CAD build for the part. Positions are in the model's coordinates, mm. Coordinates: 2 decimals unless noted, no trailing zeros. Loops run counter-clockwise (first coordinate to the right, second up) from the corner with the lowest first, then second, coordinate; pieces in that order, holes last. Notation, with made-up numbers: (47.25, -21.75) - (60.25, -21.75) arc R21 cw to (60.25, 6.25) - close; hole circle Ø11 at (12, 64.25). An arc over 180 degrees is marked (long way). Put each result on its own line as item: value.
```python
from build123d import *

# Parameters (mm, degrees)
F0_R     = 11
F1_DEPTH = 9
F2_R     = 1.5
F3_SIZE  = 1


with BuildPart() as f1:
    # F0 (on Top) → F1 (new body)
    with BuildSketch(Plane.XY):
        with BuildLine():
            ThreePointArc((-8.613839, 14.656117), (-15.257844, 12.618509), (-22.107143, 13.793993))
            ThreePointArc((-22.107143, 13.793993), (-43, 0), (-22.107143, -13.793993))
            ThreePointArc((-22.107143, -13.793993), (-15.257844, -12.618509), (-8.613839, -14.656117))
            ThreePointArc((-8.613839, -14.656117), (0, -17), (8.613839, -14.656117))
            ThreePointArc((8.613839, -14.656117), (15.257844, -12.618509), (22.107143, -13.793993))
            ThreePointArc((22.107143, -13.793993), (43, 0), (22.107143, 13.793993))
            ThreePointArc((22.107143, 13.793993), (15.257844, 12.618509), (8.613839, 14.656117))
            ThreePointArc((8.613839, 14.656117), (0, 17), (-8.613839, 14.656117))
        make_face()
        with Locations((-28, 0)):
            Circle(F0_R, mode=Mode.SUBTRACT)
        Circle(F0_R, mode=Mode.SUBTRACT)
        with Locations((28, 0)):
            Circle(F0_R, mode=Mode.SUBTRACT)
    extrude(amount=F1_DEPTH)

    # F2
    f2_edges = [f1.edges().sort_by_distance(p)[0] for p in [
        (0, 17, 0),
        (0, 17, 9),
    ]]
    fillet(f2_edges, radius=F2_R)

    # F3
    f3_edges = [f1.edges().sort_by_distance(p)[0] for p in [
        (-17, 0, 4.5),
        (-39, 0, 0),
        (-39, 0, 9),
        (11, 0, 4.5),
        (-11, 0, 0),
        (-11, 0, 9),
        (39, 0, 4.5),
        (17, 0, 0),
        (17, 0, 9),
    ]]
    chamfer(f3_edges, length=F3_SIZE)


solid = f1.part
```
Q1. Slice it at C-C, the plane y = -6. State how many separate pieces and enclosed holes the cut face has, then the cut area to 3 significant figures.
Determined:
separate pieces: 4
enclosed holes: 0
area: 244 mm2
Q2. Slice it at A-A, the plane x = 0. Give the cut face in (y, z), then the cut area to 3 significant figures.
Determined:
outline: (-17, 1.5) arc R1.5 ccw to (-15.5, 0) - (-12, 0) - (-11, 1) - (-11, 8) - (-12, 9) - (-15.5, 9) arc R1.5 ccw to (-17, 7.5) - close; (11, 1) - (12, 0) - (15.5, 0) arc R1.5 ccw to (17, 1.5) - (17, 7.5) arc R1.5 ccw to (15.5, 9) - (12, 9) - (11, 8) - close
area: 104 mm2
Q3. Slice it at B-B, the plane z = 2.25. Give the cut face in (x, y).
Determined:
outline: (-22.11, -13.79) arc R15 cw to (-8.61, -14.66) arc R17 ccw to (8.61, -14.66) arc R15 cw to (22.11, -13.79) arc R15 ccw (long way) to (22.11, 13.79) arc R15 cw to (8.61, 14.66) arc R17 ccw to (-8.61, 14.66) arc R15 cw to (-22.11, 13.79) arc R15 ccw (long way) to start; hole circle Ø22 at (-28, 0); hole circle Ø22 at (0, 0); hole circle Ø22 at (28, 0)
Q4. Pin check, flat tips, straight feed: pin 1 Ø2 at (y, z) = (4.5, 7) entering from +X; pin 2 Ø20 at (x, y) = (28, 0) entering from -Z; pin 3 Ø3 at (y, z) = (-12.5, 5.5) entering from -X; pin 4 Ø3 at (x, z) = (-8, 1.5) entering from +Y. Stop position of each tip, or through.
Determined:
pin 1: x = 42.59
pin 2: through
pin 3: x = -38.2
pin 4: y = 15.71
Q5. Mould opens along Y. For faces 1 (the cylindrical face through (38.161, -4.213, 4.451)), 2 (the cylindrical face through (0, 17, 4)), 3 (the flat face through (-12.5, 1.2, 9)) say: +Y half, -Y half, draft (parallel to the pull), parting line (faces both ways), or undercut.
Determined:
face 1: undercut
face 2: +Y half
face 3: draft
Q6. Wall check: L1, parallel to X at y = -3.5, z = 1; L2, parallel to X at y = 10, z = 5.75; L3, parallel to Y at x = 28, z = 5.25. Give the ranges that are in metal, low to high. Write a range as from..to.
Determined:
L1: -42.5..-38.43, -17.57..-10.43, 10.43..17.57, 38.43..42.5
L2: -39.18..-32.58, -23.42..-4.58, 4.58..23.42, 32.58..39.18
L3: -15..-11, 11..15
